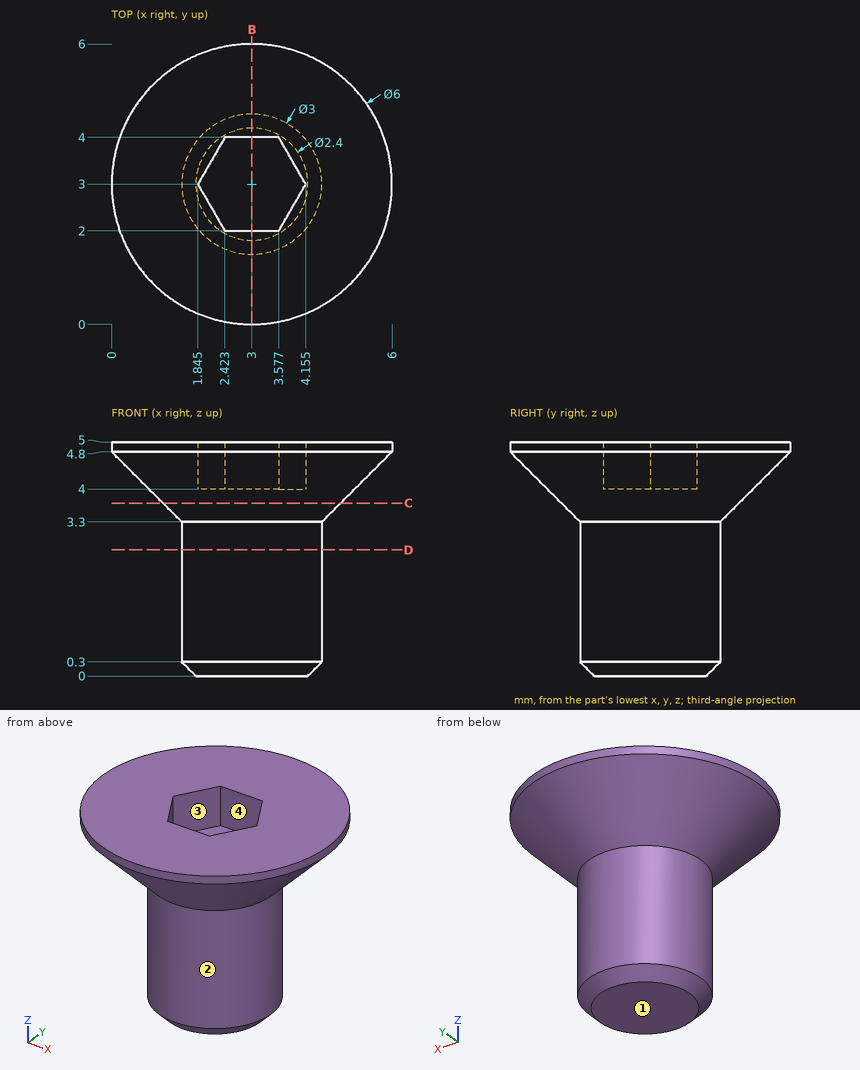
The drawing under review shows one solid part. Ordinate dimensions are in mm from its lowest x, y, z. Round coordinates to 2 decimals unless told otherwise and drop trailing zeros. Loops run counter-clockwise (first coordinate to the right, second up) from the corner with the lowest first, then second, coordinate; pieces in that order, holes last. Notation, with made-up numbers: (37.25, -36.5) - (91.25, -36.5) arc R33 ccw to (91.25, -4.5) - close; hole circle Ø11 at (14.5, 71.25). An arc over 180 degrees is marked (long way). Use a Markdown table: item, result. Add a question column.
Q1. For probe 1 along Z at (x, y) = (5.05, 1.95) (1 decimal); probe 2 along X at (y, z) = (1.15, 3.95) (1 decimal); probe 3 along Z at (x, y) = (5.75, 3.6) (1 decimal), list the stretches that pass through material, from the lowest coordinate up.
Q2. Insertion check: pin 1 Ø1.5 at (x, z) = (5.5, 2) entering from +Y; pin 2 Ø3 at (y, z) = (3, 3) entering from +X. Each pin has a flat end and moves straight along its axis. Give the tip position at first contact, or say it passes through.
Q3. Add section B-B (x = 3). State the section outline as (y, z) points.
Q4. The part is to be moulded in two halves that separate along Y. For the marked faces 1, 2, 3 and 4, say which applies: pulls with the +Y half, pulls with the -Y half, needs draft (parallel to the pull), parting line crosses it, or undercut.
Q5. Add section D-D (z = 2.7). State the section outline as (x, y) points.
Q6. Add section C-C (z = 3.7). State the section outline as (x, y) points.
Worked answers:
| question | item | result |
|---|---|---|
| 1 | probe 1 | 4.1 to 5 |
| 1 | probe 2 | 1.9 to 4.1 |
| 1 | probe 3 | 4.6 to 5 |
| 2 | pin 1 | through |
| 2 | pin 2 | x = 5.7 |
| 3 | outline | (0, 4.8) - (1.5, 3.3) - (1.5, 0.3) - (1.8, 0) - (4.2, 0) - (4.5, 0.3) - (4.5, 3.3) - (6, 4.8) - (6, 5) - (4, 5) - (4, 4) - (2, 4) - (2, 5) - (0, 5) - close |
| 4 | face 1 | needs draft |
| 4 | face 2 | parting line crosses it |
| 4 | face 3 | undercut |
| 4 | face 4 | undercut |
| 5 | outline | circle Ø3 at (3, 3) |
| 6 | outline | circle Ø3.8 at (3, 3) |
